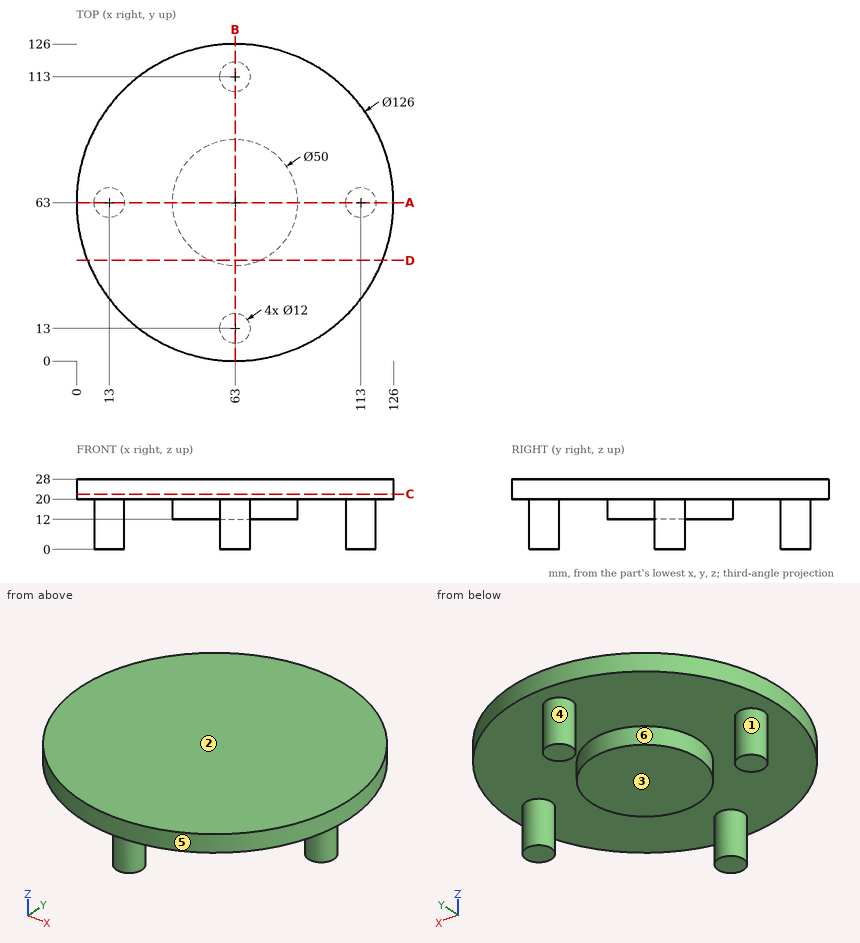
Design review of the part shown in the three views and the two pictorial views. Dimensions are in mm from the part's minimum x, y and z. A direction names the side the tool comes from. Coordinates: 2 decimals unless noted, no trailing zeros. Order: outer loops, then holes, each group sorted by start corner. A loop starts at its lowest first (then second) coordinate and runs counter-clockwise, first axis right, second up.
Item 1: Take a section at A-A, the plane y = 63. Write out the cut boundary in (x, z), then the cut area to 3 significant figures.
Item 2: For line 1 (Y direction, x = 63.5, z = 19) (3 decimals); line 2 (Y direction, x = 63.5, z = 3.25); line 3 (Z direction, x = 88.5, y = 85.5), list the stretches that pass through material, from the lowest coordinate up.
Item 3: For the marked faces 5 and 6, list the 3-axis set-ups (+Z, -Z, +X, -X, +Y, -Y) from which the entire face can be reached by the end or side of a thin tool; tool diameter is ignored.
Item 4: Take a section at C-C, the plane z = 22. Write out the cut boundary in (x, y), then the cut area to 3 significant figures.
Item 5: For pin 1 Ø12 at (x, z) = (108.5, 19) entering from +Y; pin 2 Ø5 at (x, y) = (96.5, 55.5) entering from -Z; pin 3 Ø8 at (x, z) = (33, 24) entering from -Y, all flat-tipped, find the tip position at first contact; note any pin that passes through.
Item 6: Take a section at D-D, the plane y = 40. Write out the cut boundary in (x, z), then the cut area to 3 significant figures.
Item 7: The part is to be moulded in two halves that separate along X. For the marked faces 1, 2, 3 and 4, say which applies: pulls with the +X half, pulls with the -X half, needs draft (parallel to the pull), parting line crosses it, or undercut.
The answers:
1. outline: (0, 20) - (7, 20) - (7, 0) - (19, 0) - (19, 20) - (38, 20) - (38, 12) - (88, 12) - (88, 20) - (107, 20) - (107, 0) - (119, 0) - (119, 20) - (126, 20) - (126, 28) - (0, 28) - close
1. area: 1,890 mm2
2. line 1: y = 7.021 to 18.979, 38.005 to 87.995, 107.021 to 118.979
2. line 2: y = 7.02 to 18.98, 107.02 to 118.98
2. line 3: z = 20 to 28
3. face 5: +Z, -Z
3. face 6: -Z
4. outline: circle Ø126 at (63, 63)
4. area: 12,500 mm2
5. pin 1: stops at y = 112.01
5. pin 2: stops at z = 20
5. pin 3: stops at y = 5.62
6. outline: (4.35, 20) - (53.2, 20) - (53.2, 12) - (72.8, 12) - (72.8, 20) - (121.65, 20) - (121.65, 28) - (4.35, 28) - close
6. area: 1,100 mm2
7. face 1: undercut
7. face 2: needs draft
7. face 3: undercut
7. face 4: parting line crosses it
